Could you check a few things on this drawing? It's one solid part, dimensions in mm from its lowest x, y, z. A direction names the side the tool comes from. Give positions to 0.01 mm unless a question says otherwise; leave off trailing zeros. Loops run counter-clockwise (first coordinate to the right, second up) from the corner with the lowest first, then second, coordinate; pieces in that order, holes last. Notation, with made-up numbers: M 2.5,7.25 L 23.5,7.25 A27 cw 23.5,24.25 Z; hole C 10.25,88.5 d6. An arc over 180 degrees is marked long. Answer in a Markdown table with one row per item. Add a question column.
1. I'm going to push flat-ended pins straight in: pin 1 Ø4 at (x, y) = (67.5, 32) entering from -Z; pin 2 Ø12 at (y, z) = (67, 81) entering from +X; pin 3 Ø2 at (x, y) = (67.5, 85) entering from +Z. Where does each tip first touch, or does it pass through?
2. If we section it at D-D on y = 4: List the corners of the cut face in (x, z) for me, then the cut area to 3 significant figures.
3. I need wall thicknesses on line 1 along Z through (x, y) = (93, 90.5); line 2 along Z through (x, y) = (27, 90); line 3 along Y through (x, z) = (119.5, 100). Which ranges of each line are inside material? Lowest first, please. Write a range as from..to.
4. If we section it at B-B on z = 4: List the corners of the cut face in (x, y) for me, then the cut area to 3 significant figures.
5. Thinking about a two-plate mould opening in Z: for the marked faces 6, 7 and 8, which applies, released by +Z, released by -Z, zero draft, split by the parting line, or undercut?
6. If we section it at C-C on y = 85: List the corners of the cut face in (x, z) for me.
7. Which directions (+Z, -Z, +X, -X, +Y, -Y) give clear straight access to the entire face, cutting with the end or side of a thin tool? Please do the marked faces 1, 2, 3, 4 and 5.
8. If we section it at A-A on x = 105: List the corners of the cut face in (y, z) for me, then the cut area to 3 significant figures.
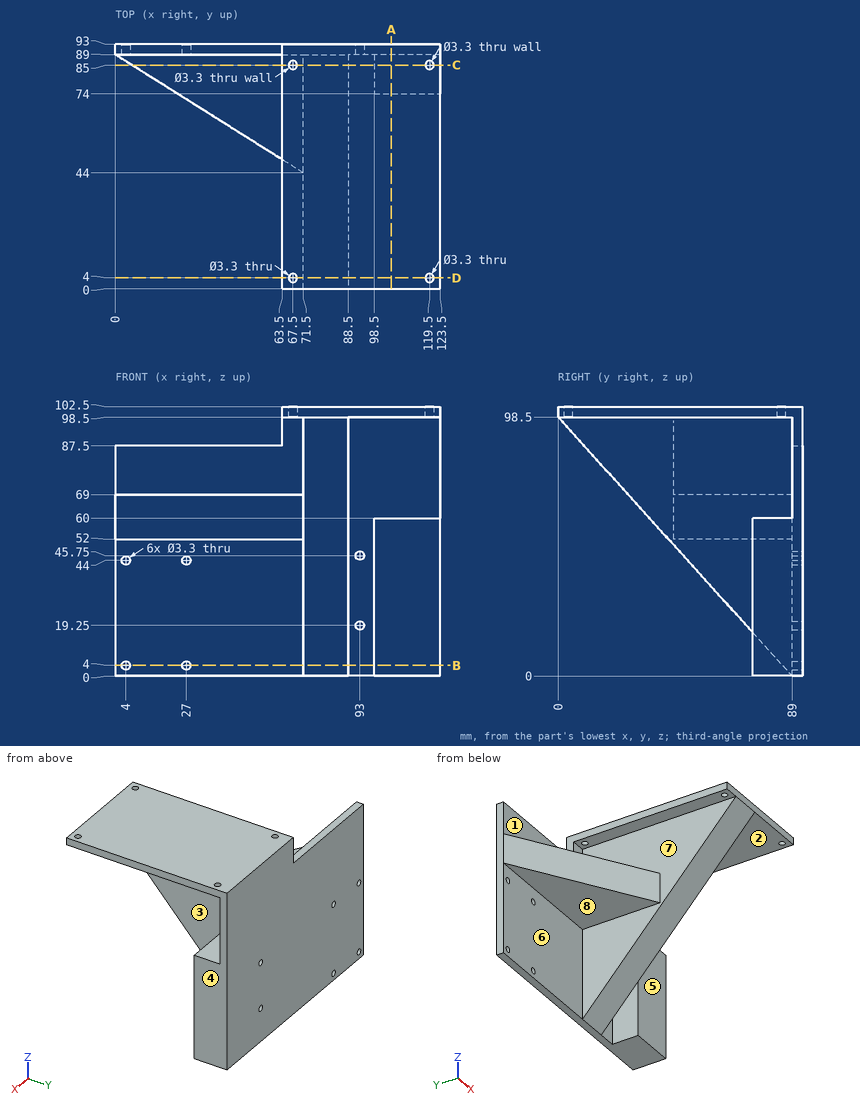
Results:
| question | item | result |
|---|---|---|
| 1 | pin 1 | z = 98.5 |
| 1 | pin 2 | x = 88.5 |
| 1 | pin 3 | z = 69 |
| 2 | outline | M 63.5,98.5 L 65.85,98.5 L 65.85,102.5 L 63.5,102.5 Z; M 69.15,98.5 L 71.5,98.5 L 71.5,94.07 L 88.5,94.07 L 88.5,98.5 L 117.85,98.5 L 117.85,102.5 L 69.15,102.5 Z; M 121.15,98.5 L 123.5,98.5 L 123.5,102.5 L 121.15,102.5 Z |
| 2 | area | 289 mm2 |
| 3 | line 1 | 0..17.6, 20.9..44.1, 47.4..102.5 |
| 3 | line 2 | 0..2.35, 5.65..42.35, 45.65..87.5 |
| 3 | line 3 | 0..2.35, 5.65..83.35, 86.65..93 |
| 4 | outline | M 0,89 L 2.35,89 L 2.35,93 L 0,93 Z; M 5.65,89 L 25.35,89 L 25.35,93 L 5.65,93 Z; M 28.65,89 L 71.5,89 L 71.5,85.39 L 88.5,85.39 L 88.5,89 L 98.5,89 L 98.5,74 L 123.5,74 L 123.5,93 L 28.65,93 Z |
| 4 | area | 904 mm2 |
| 5 | face 6 | zero draft |
| 5 | face 7 | undercut |
| 5 | face 8 | released by -Z |
| 6 | outline | M 6.36,52 L 71.5,52 L 71.5,4.43 L 88.5,4.43 L 88.5,98.5 L 117.85,98.5 L 117.85,102.5 L 69.15,102.5 L 69.15,98.5 L 71.5,98.5 L 71.5,69 L 6.36,69 Z; M 63.5,98.5 L 65.85,98.5 L 65.85,102.5 L 63.5,102.5 Z; M 98.5,0 L 123.5,0 L 123.5,60 L 98.5,60 Z; M 121.15,98.5 L 123.5,98.5 L 123.5,102.5 L 121.15,102.5 Z |
| 7 | face 1 | -X, -Y |
| 7 | face 2 | +X, -Y |
| 7 | face 3 | -Z, -Y |
| 7 | face 4 | +Z, -Z, +X, +Y, -Y |
| 7 | face 5 | -Z, +X, -Y |
| 8 | outline | M 0,98.5 L 89,98.5 L 89,60 L 74,60 L 74,0 L 93,0 L 93,102.5 L 0,102.5 Z |
| 8 | area | 1,670 mm2 |
